Check sheet for the modelled part. Datum: model origin and axes. Units: mm. Face numbers are marked on the shaded views. A direction names the side the tool comes from. Round coordinates to 2 decimals unless told otherwise and drop trailing zeros. Loops run counter-clockwise (first coordinate to the right, second up) from the corner with the lowest first, then second, coordinate; pieces in that order, holes last. Notation, with made-up numbers: M 38,-15.75 L 55,-15.75 A11 cw 55,-2.75 Z; hole C -19.5,-7.5 d8. An arc over 180 degrees is marked long. Write item = value, one per line. Start each with the question number.
(1) Scan lines: L1, parallel to Y at x = 0, z = 2.8; L2, parallel to Y at x = 0, z = 0.75; L3, parallel to Z at x = 17, y = -12. Record each from-to range of solid material in increasing order. Write a range as from..to.
(2) Set-up check for the marked faces 4 and 5: record each of +Z, -Z, +X, -X, +Y, -Y from which the full face is reachable in a straight line by a thin tool's end or side.
(3) Cross-section at B-B on z = 9.5. Record the boundary of the cut face in (x, y), plus the area to 3 significant figures.
(4) Cross-section at A-A on y = 1.5. State how many separate pieces and enclosed holes the cut face has, plus the area to 3 significant figures.
(5) Go/stop test with flat-tipped pins: P1, Ø14.5, axis at x = 0, y = 21, coming from the -Z side; P2, Ø18.5, axis at x = 14, y = -1, coming from the +Z side; P3, Ø5.5, axis at x = 0, y = 21, coming from the +Z side; P4, Ø4.5, axis at y = -8, z = 3, coming from the -X side. Record where each tip stops, or that it passes through.
(6) Mould release check, pull along Z, two halves, no side actions. Record for the marked faces 1, 2 and 3: pulls with the +Z half, pulls with the -Z half, needs draft (parallel to the pull), parting line crosses it, or undercut.
from build123d import *

# Parameters (mm, degrees)
SKETCH1_W                = 15
SKETCH1_H                = 31
SKETCH1_R                = 3
BOSS_EXTRUDE1_DEPTH      = 4
SKETCH2_R                = 4.5
CUT_EXTRUDE1_DEPTH       = 2
CHAMFER1_SIZE            = 2
BOSS_EXTRUDE3_DEPTH      = 4
SKETCH4_R                = 13.5
SKETCH4_R_2              = 12
BOSS_EXTRUDE4_DEPTH      = 51.220242393
BOSS_EXTRUDE5_REACH      = 79.695
BOSS_EXTRUDE5_END_RADIUS = 13.5


with BuildPart() as part:
    # Sketch1 → Boss-Extrude1 (new body)
    with BuildSketch(Plane.XY):
        with Locations((0, 10.5)):
            Rectangle(SKETCH1_W, SKETCH1_H)
        Circle(SKETCH1_R, mode=Mode.SUBTRACT)
        with Locations((0, 21)):
            Circle(SKETCH1_R, mode=Mode.SUBTRACT)
    extrude(amount=BOSS_EXTRUDE1_DEPTH)

    # Sketch2 → Cut-Extrude1 (cut)
    with BuildSketch(Plane.XY.offset(4)):
        with Locations((0, 21)):
            Circle(SKETCH2_R)
        Circle(SKETCH2_R)
    extrude(amount=-CUT_EXTRUDE1_DEPTH, mode=Mode.SUBTRACT)

    # Chamfer1
    chamfer1_edges = [part.edges().sort_by_distance(p)[0] for p in [
        (-7.5, -5, 2),
        (-7.5, 26, 2),
    ]]
    chamfer(chamfer1_edges, length=CHAMFER1_SIZE)

    # Sketch3 → Boss-Extrude3 (add)
    with BuildSketch(Plane.XY.offset(4)):
        Polygon((1.423063068, -5), (7.5, -5), (7.5, 26), (36.782487596, 26), (54.611806547, 8.17068105), (41.441125497, -5), (18.393625817, -28.04749968), (1.423063068, -11.076936932), align=None)
    extrude(amount=-BOSS_EXTRUDE3_DEPTH)



with BuildPart() as body_2:
    # Sketch4 → Boss-Extrude4 (new body)
    with BuildSketch(Plane(origin=(31.391243798, 31.391243798, 0), x_dir=(0, 0, -1), z_dir=(0.7071067811865465, 0.7071067811865487, 0))):
        with Locations(Location((-37, -20.231602431, 0), (0, 0, 90))):
            Circle(SKETCH4_R)
        with Locations(Location((-37, -20.231602431, 0), (0, 0, 90))):
            Circle(SKETCH4_R_2, mode=Mode.SUBTRACT)
    extrude(amount=-BOSS_EXTRUDE4_DEPTH)


with BuildPart() as part_1:
    add(part.part)

    add(body_2.part)  # Boss-Extrude5 merges body 2
    # Boss-Extrude5: up to this cylinder (the profile starts outside it)
    boss_extrude5_end = Plane(origin=(27.737015773, -0.874790773, 37), z_dir=(0.7071067811865465, 0.7071067811865487, 0)) * Cylinder(BOSS_EXTRUDE5_END_RADIUS, 187.39, mode=Mode.PRIVATE)
    # Sketch5 → Boss-Extrude5 (add, up to the surface)
    with BuildSketch(Plane.XY.offset(4), mode=Mode.PRIVATE) as boss_extrude5_sk1:
        Polygon((1.423063068, -11.076936932), (36.782487596, 26), (54.611806547, 8.17068105), (18.393625817, -28.04749968), align=None)
    boss_extrude5_tool1 = extrude(boss_extrude5_sk1.sketch, amount=BOSS_EXTRUDE5_REACH, mode=Mode.PRIVATE) - boss_extrude5_end
    add(boss_extrude5_tool1.solids().sort_by_distance((27.949939, -1.087714, 4))[0])


solid = part_1.part
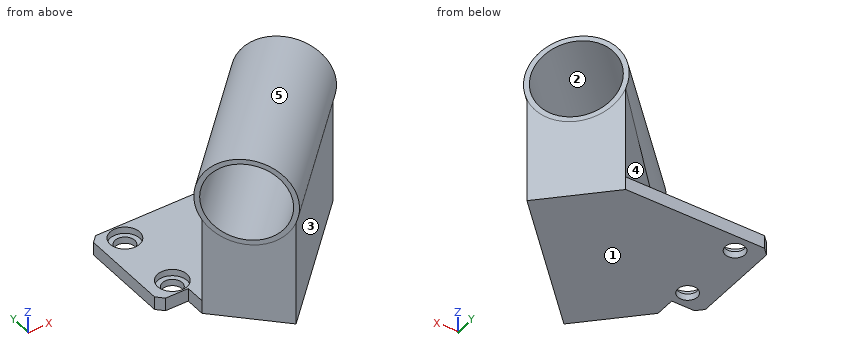
Result:
q1.L1 = -5..-4.5, 4.5..16.5, 25.5..26
q1.L2 = -5..-3, 3..18, 24..26
q1.L3 = 0..25, 49..50.5
q2.face_4 = -X, +Y
q2.face_5 = none
q3.outline = M 1.42,-11.08 L 18.39,-28.05 L 54.61,8.17 L 36.78,26 Z
q3.area = 1,260 mm^2
q4.separate_pieces = 2
q4.enclosed_holes = 1
q4.area = 1,110 mm^2
q5.P1 = 0
q5.P2 = 50.49
q5.P3 = through
q5.P4 = 1.42
q6.face_1 = pulls with the -Z half
q6.face_2 = undercut
q6.face_3 = needs draft
